Can you work these out from the model? Positions are in its coordinate system, mm. A direction names the side the tool comes from. Give positions to 0.01 mm unless a question says otherwise; leave off trailing zeros. Write each loop counter-clockwise with the first axis right and the second up, starting at its lowest first coordinate (ties: lowest second). Pieces come first, ordered by that corner, then holes.
from build123d import *

# Parameters (mm, degrees)
F1_DEPTH = 5
F2_T     = 2


with BuildPart() as f1:
    # F0 (on Top) → F1 (new body)
    with BuildSketch(Plane.XY):
        Polygon((0, 20), (-20, 20), (-20, -20), (20, -20), (20, 0), (0, 0), align=None)
    extrude(amount=F1_DEPTH)

    # F2
    f2_openings = [f1.faces().sort_by_distance(p)[0] for p in [
        (-3.333333, -3.333333, 5),
        (20, -10, 2.5),
        (-10, 20, 2.5),
    ]]
    offset(amount=F2_T, openings=f2_openings, kind=Kind.INTERSECTION)


solid = f1.part
(1) For faces 4 (the face through (11, 2, 1)), 5 (the face through (-21, -10, 5)), 6 (the face through (20, -10, -1)), 7 (the face through (0, 10, 2)), 8 (the face through (10, 0, 2)), which set-ups out of +Z, -Z, +X, -X, +Y, -Y let a thin tool reach every point of the face, with its end or its side?
Returned:
face 4: +Z, -Z, +X, +Y
face 5: +Z, +X, -X, +Y, -Y
face 6: +Z, -Z, +X, +Y, -Y
face 7: +Z, +Y
face 8: +Z, +X
(2) If we mould it in two halves opening along Y, with no side actions, what happens to faces 1 (the face through (-1, -22, 1)), 2 (the face through (-5, -4, 0)), 3 (the face through (-22, -1, 1))? For each: +Y half, -Y half, draft (parallel to the pull), parting line (faces both ways), or undercut.
Returned:
face 1: -Y half
face 2: undercut
face 3: draft
(3) If I drill on L1, parallel to X at y = 5.5, z = 4; L2, parallel to Y at x = -4, z = 1.25; L3, parallel to Z at x = -12, y = -3, over which ranges is the centre line in solid material (lowest first)?
Returned:
L1: x = -22 to -20, 0 to 2
L2: y = -22 to -20
L3: z = -2 to 0
(4) Imagine slicing it at A-A, the plane z = 2.75. Write out the boundary of the cut face in (x, y).
Returned:
outline: (-22, -22) - (20, -22) - (20, -20) - (-20, -20) - (-20, 20) - (-22, 20) - close; (0, 0) - (20, 0) - (20, 2) - (2, 2) - (2, 20) - (0, 20) - close
(5) Imagine slicing it at B-B, the plane y = 14. Write out the boundary of the cut face in (x, z), plus the area to 3 significant figures.
Returned:
outline: (-22, -2) - (2, -2) - (2, 5) - (0, 5) - (0, 0) - (-20, 0) - (-20, 5) - (-22, 5) - close
area: 68.0 mm2
(6) Will these pins go through, and if not, where does the flat tip stop? P1, Ø3.5, axis at y = 12.5, z = 3, coming from the +X side; P2, Ø2, axis at x = -9, y = -6, coming from the +Z side; P3, Ø1.5, axis at x = -2, z = 0.5, coming from the +Y side; P4, Ø2, axis at x = 13.5, z = 2.5, coming from the +Y side.
Returned:
P1: stops at x = 2
P2: stops at z = 0
P3: stops at y = 20
P4: stops at y = 2
(7) Imagine slicing it at D-D, the plane z = -1. Write out the boundary of the cut face in (x, y).
Returned:
outline: (-22, -22) - (20, -22) - (20, 2) - (2, 2) - (2, 20) - (-22, 20) - close
(8) Imagine slicing it at C-C, the plane x = -13. Write out the boundary of the cut face in (y, z).
Returned:
outline: (-22, -2) - (20, -2) - (20, 0) - (-20, 0) - (-20, 5) - (-22, 5) - close
